from build123d import *

# Parameters (mm, degrees)
F0_R     = 7.1
F1_DEPTH = 12.7
F2_R     = 1.75
F3_DEPTH = 0.5


# Not quite as in the source:
# - ends of sketch curves that miss each other by under 0.0002 mm in the source are joined


with BuildPart() as f1:
    # F0 (on Front) → F1 (new body)
    with BuildSketch(Plane.XZ):
        Circle(F0_R)
    extrude(amount=F1_DEPTH)

    # F2 (on Front) → F3 (join)
    with BuildSketch(Plane.XZ):
        with BuildLine():
            Line((10.246950766, -3.25), (11.9, -3.25))
            ThreePointArc((11.9, -3.25), (15.15, 0), (11.9, 3.25))
            Line((11.9, 3.25), (10.2469522811, 3.25))
            ThreePointArc((10.2469522811, 3.25), (6.3492135874, 8.6746768166), (0, 10.7500014442))
            ThreePointArc((0, 10.7500014442), (-6.3492135874, 8.6746768166), (-10.2469522811, 3.25))
            Line((-10.2469522811, 3.25), (-11.9, 3.249995223))
            Line((-11.9, 3.249995223), (-11.9055723148, 3.249995223))
            ThreePointArc((-11.9055723148, 3.249995223), (-15.1499988057, -0.0027861584), (-11.9, -3.25))
            Line((-11.9, -3.25), (-10.246950766, -3.25))
            ThreePointArc((-10.246950766, -3.25), (-6.3492125496, -8.6746757864), (0, -10.75))
            ThreePointArc((0, -10.75), (6.3492125496, -8.6746757864), (10.246950766, -3.25))
        make_face()
        with Locations((-11.9, 0)):
            Circle(F2_R, mode=Mode.SUBTRACT)
        with Locations((11.9, 0)):
            Circle(F2_R, mode=Mode.SUBTRACT)
    extrude(amount=F3_DEPTH)


solid = f1.part
Can you work these out from the model? Positions are in its coordinate system, mm. A direction names the side the tool comes from. Give positions to 0.01 mm unless a question says otherwise; leave off trailing zeros. Write each loop counter-clockwise with the first axis right and the second up, starting at its lowest first coordinate (ties: lowest second). Pieces come first, ordered by that corner, then holes. Notation, with made-up numbers: M 9.5,-13 L 26.5,-13 A16 ccw 26.5,0 Z; hole C -36.5,18 d10. An arc over 180 degrees is marked long. Answer in a Markdown table with one row per item. Add a question column.
Item 1: On a 3-axis mill with a long thin cutter (end or side, diameter ignored), from which of +Z, -Z, +X, -X, +Y, -Y can I reach the whole of each face in a straight line? I mean faces 1 (the flat face through (0, 0, 0)), 2 (the cylindrical face through (-0.92, -6.51, 7.04)). Say none if no direction works.
Item 2: For pin 1 Ø8 at (x, z) = (-12, -1) entering from -Y; pin 2 Ø1.5 at (x, y) = (-5, -2) entering from -Z; pin 3 Ø6 at (x, z) = (5.5, -7) entering from +Y; pin 4 Ø6 at (x, y) = (7.5, -6) entering from -Z, each with a flat end and sliding along its axis, tell me the tip position at first contact or that it passes through.
Item 3: Imagine slicing it at A-A, the plane z = 0. Write out the boundary of the cut face in (x, y), plus the area to 3 significant figures.
Item 4: Imagine slicing it at B-B, the plane x = 4. Write out the boundary of the cut face in (y, z), plus the area to 3 significant figures.
Item 5: Imagine slicing it at D-D, the plane z = -5.25. Write out the boundary of the cut face in (x, y).
Item 6: Imagine slicing it at C-C, the plane y = -11.25. Write out the boundary of the cut face in (x, z).
Item 7: Please list where these lines run through material, in increasing order: L1, parallel to Z at x = 11.9, y = -0.2; L2, parallel to Z at x = 0, y = -9.75; L3, parallel to Y at x = 7, z = 5.25.
Item 8: We'd pull the mould along Z, two halves only. Please class faces 3 (the cylindrical face through (-15.15, -0.25, 0.07)), 4 (the flat face through (-7, -0.5, 3)), 5 (the cylindrical face through (13.569, -0.246, 0.526)), 6 (the cylindrical face through (-10.231, -0.246, 0.526)): released by +Z, released by -Z, zero draft, split by the parting line, or undercut.
Evaluation:
| question | item | result |
|---|---|---|
| 1 | face 1 | +Z, -Z, +X, -X, +Y |
| 1 | face 2 | -Y |
| 2 | pin 1 | stops at y = -0.5 |
| 2 | pin 2 | stops at z = -5.69 |
| 2 | pin 3 | stops at y = 0 |
| 2 | pin 4 | stops at z = -5.49 |
| 3 | outline | M -15.15,-0.5 L -13.65,-0.5 L -13.65,0 L -15.15,0 Z; M -10.15,-0.5 L -7.1,-0.5 L -7.1,-12.7 L 7.1,-12.7 L 7.1,-0.5 L 10.15,-0.5 L 10.15,0 L -10.15,0 Z; M 13.65,-0.5 L 15.15,-0.5 L 15.15,0 L 13.65,0 Z |
| 3 | area | 185 mm² |
| 4 | outline | M -12.7,-5.87 L -0.5,-5.87 L -0.5,-9.98 L 0,-9.98 L 0,9.98 L -0.5,9.98 L -0.5,5.87 L -12.7,5.87 Z |
| 4 | area | 153 mm² |
| 5 | outline | M -9.38,-0.5 L -4.78,-0.5 L -4.78,-12.7 L 4.78,-12.7 L 4.78,-0.5 L 9.38,-0.5 L 9.38,0 L -9.38,0 Z |
| 6 | outline | C 0,0 d14.2 |
| 7 | L1 | z = -3.25 to -1.75, 1.75 to 3.25 |
| 7 | L2 | z = -7.1 to 7.1 |
| 7 | L3 | y = -0.5 to 0 |
| 8 | face 3 | split by the parting line |
| 8 | face 4 | zero draft |
| 8 | face 5 | undercut |
| 8 | face 6 | undercut |
